Verification items for the finished model (mm, model axes). Coordinates: 2 decimals unless noted, no trailing zeros. Write each loop counter-clockwise with the first axis right and the second up, starting at its lowest first coordinate (ties: lowest second). Pieces come first, ordered by that corner, then holes. Notation, with made-up numbers: (69, 35) -> (78, 35) arc R13 ccw to (78, 58) -> close; hole circle Ø7 at (27.5, 12.25). An arc over 180 degrees is marked (long way). Use CSV: the item, a comma, the result in double quotes.
```python
from build123d import *

# Parameters (mm, degrees)
F0_R     = 3.25
F1_DEPTH = 68


with BuildPart() as f1:
    # F0 (on Front) → F1 (new body)
    with BuildSketch(Plane.XZ):
        with BuildLine():
            ThreePointArc((6.252197, -1.777646), (6.437751, -0.897417), (6.5, 0))
            ThreePointArc((6.5, 0), (6.437751, 0.897417), (6.252197, 1.777646))
            ThreePointArc((6.252197, 1.777646), (4.252128, 2.454967), (4.665586, 4.525739))
            ThreePointArc((4.665586, 4.525739), (3.25, 5.629165), (1.586612, 6.303385))
            ThreePointArc((1.586612, 6.303385), (0, 4.909935), (-1.586612, 6.303385))
            ThreePointArc((-1.586612, 6.303385), (-3.25, 5.629165), (-4.665586, 4.525739))
            ThreePointArc((-4.665586, 4.525739), (-4.203284, 3.963666), (-4.037769, 3.254967))
            ThreePointArc((-4.037769, 3.254967), (-4.749818, 1.923974), (-6.252197, 1.777646))
            ThreePointArc((-6.252197, 1.777646), (-6.5, 0), (-6.252197, -1.777646))
            ThreePointArc((-6.252197, -1.777646), (-4.749818, -1.923974), (-4.037769, -3.254967))
            ThreePointArc((-4.037769, -3.254967), (-4.203284, -3.963666), (-4.665586, -4.525739))
            ThreePointArc((-4.665586, -4.525739), (-3.25, -5.629165), (-1.586612, -6.303385))
            ThreePointArc((-1.586612, -6.303385), (0, -4.909935), (1.586612, -6.303385))
            ThreePointArc((1.586612, -6.303385), (3.25, -5.629165), (4.665586, -4.525739))
            ThreePointArc((4.665586, -4.525739), (4.252128, -2.454967), (6.252197, -1.777646))
        make_face()
        Circle(F0_R, mode=Mode.SUBTRACT)
    extrude(amount=F1_DEPTH)


solid = f1.part
```
1) Gauge pin test, flat end, axial feed: pin 1 (1.5 mm diameter, centred on y = -45.5, z = -1, fed in from -X). Record the tip position at first contact, or that the pin passes through.
Return value:
pin 1,"x = -6.5"
2) Mould release check, pull along X, two halves, no side actions. Record for faces 1 (the cylindrical face through (4.24, -33.52, -2.48)), 2 (the cylindrical face through (-3.23, -33.52, 5.64)), 3 (the cylindrical face through (3.3, -33.5, 5.6)): released by +X, released by -X, zero draft, split by the parting line, or undercut.
Return value:
face 1,"undercut"
face 2,"released by -X"
face 3,"released by +X"
3) Scan lines: L1, parallel to Z at x = 0, y = -51; L2, parallel to Z at x = 4.5, y = -50.5; L3, parallel to X at y = -24.5, z = -5.5. Record each from-to range of solid material in increasing order.
Return value:
L1,"-4.91 to -3.25, 3.25 to 4.91"
L2,"-4.69 to -4.38, -2.13 to 2.13, 4.38 to 4.69"
L3,"-3.46 to -1.24, 1.24 to 3.46"
4) Cross-section at A-A (y = -7). Record the boundary of the cut face in (x, z), plus the area to 3 significant figures.
Return value:
outline,"(-6.25, -1.78) arc R1.6 cw to (-4.04, -3.25) arc R1.6 cw to (-4.67, -4.53) arc R6.5 ccw to (-1.59, -6.3) arc R1.6 cw to (1.59, -6.3) arc R6.5 ccw to (4.67, -4.53) arc R1.6 cw to (6.25, -1.78) arc R6.5 ccw to (6.5, 0) arc R6.5 ccw to (6.25, 1.78) arc R1.6 cw to (4.67, 4.53) arc R6.5 ccw to (1.59, 6.3) arc R1.6 cw to (-1.59, 6.3) arc R6.5 ccw to (-4.67, 4.53) arc R1.6 cw to (-4.04, 3.25) arc R1.6 cw to (-6.25, 1.78) arc R6.5 ccw to start; hole circle Ø6.5 at (0, 0)"
area,"76.9 mm2"
5) Cross-section at B-B (x = 0). Record the boundary of the cut face in (y, z).
Return value:
outline,"(-68, -4.91) -> (0, -4.91) -> (0, -3.25) -> (-68, -3.25) -> close; (-68, 3.25) -> (0, 3.25) -> (0, 4.91) -> (-68, 4.91) -> close"
